```python
from build123d import *

# Parameters (mm, degrees)
SKETCH1_R           = 2.65
SKETCH1_W           = 1
SKETCH1_H           = 8
SKETCH1_W_2         = 14
BOSS_EXTRUDE1_DEPTH = 5
CHAMFER1_SIZE       = 3
BOSS_EXTRUDE2_DEPTH = 4
SKETCH3_R           = 5
CUT_EXTRUDE1_DEPTH  = 11.5


with BuildPart() as part:
    # Sketch1 → Boss-Extrude1 (new body)
    with BuildSketch(Plane.XY):
        Polygon((-14, -2.5), (-14, 0), (-15, 0), (-15, 8), (-14, 8), (-14, 10.5), (-27.5, 10.5), (-27.5, -2.5), align=None)
        with Locations((-21, 4)):
            Circle(SKETCH1_R, mode=Mode.SUBTRACT)
        with Locations((-14.5, 4)):
            Rectangle(SKETCH1_W, SKETCH1_H)
        with Locations((-7, 4)):
            Rectangle(SKETCH1_W_2, SKETCH1_H)
        with Locations((7, 4)):
            Rectangle(SKETCH1_W_2, SKETCH1_H)
        with Locations((14.5, 4)):
            Rectangle(SKETCH1_W, SKETCH1_H)
        Polygon((15, 8), (15, 0), (14, 0), (14, -2.5), (27.5, -2.5), (27.5, 10.5), (14, 10.5), (14, 8), align=None)
        with Locations((21, 4)):
            Circle(SKETCH1_R, mode=Mode.SUBTRACT)
    extrude(amount=BOSS_EXTRUDE1_DEPTH)

    # Chamfer1
    chamfer1_edges = [part.edges().sort_by_distance(p)[0] for p in [
        (27.5, 10.5, 2.5),
        (27.5, -2.5, 2.5),
        (-27.5, -2.5, 2.5),
        (-27.5, 10.5, 2.5),
    ]]
    chamfer(chamfer1_edges, length=CHAMFER1_SIZE)

    # Sketch2 → Boss-Extrude2 (add, symmetric)
    with BuildSketch(Plane(origin=(0, 4, 0), x_dir=(1, 0, 0), z_dir=(0, 1, 0))):
        with BuildLine():
            Line((-14, -5), (-14, 10))
            ThreePointArc((-14, 10), (0, 24), (14, 10))
            Line((14, 10), (14, -5))
            Line((14, -5), (-14, -5))
        make_face()
    extrude(amount=BOSS_EXTRUDE2_DEPTH, both=True)

    # Sketch3 → Cut-Extrude1 (cut, through all)
    with BuildSketch(Plane(origin=(0, 8, 0), x_dir=(1, 0, 0), z_dir=(0, 1, 0))):
        with Locations((0, 10)):
            Circle(SKETCH3_R)
    extrude(amount=-CUT_EXTRUDE1_DEPTH, mode=Mode.SUBTRACT)


solid = part.part
```
For this review, take the finished solid that the model builds, in its own axes (mm). A direction names the side the tool comes from. Give positions to 0.01 mm unless a question says otherwise; leave off trailing zeros. Write each loop counter-clockwise with the first axis right and the second up, starting at its lowest first coordinate (ties: lowest second). Pieces come first, ordered by that corner, then holes. Notation, with made-up numbers: M 52,-5.75 L 101,-5.75 A30 ccw 101,32.25 Z; hole C 49,35.5 d11. An arc over 180 degrees is marked long. One line per item, written item: value.
1) For P1, Ø6.5, axis at y = 3, z = -5.5, coming from the -X side; P2, Ø12, axis at x = 8, z = -2.5, coming from the +Y side; P3, Ø1.5, axis at y = -0.5, z = -1, coming from the +X side; P4, Ø1, axis at y = 9, z = -2, coming from the -X side, all flat-tipped, find the tip position at first contact; note any pin that passes through.
Results are:
P1: stops at x = -14
P2: stops at y = 8
P3: stops at x = 14
P4: passes through
2) Take a section at D-D, the plane x = 21. Write out the cut boundary in (y, z).
Results are:
outline: M -2.5,0 L 1.35,0 L 1.35,5 L -2.5,5 Z; M 6.65,0 L 10.5,0 L 10.5,5 L 6.65,5 Z
3) Take a section at A-A, the plane x = 0. Write out the cut boundary in (y, z).
Results are:
outline: M 0,-24 L 8,-24 L 8,-15 L 0,-15 Z; M 0,-5 L 8,-5 L 8,5 L 0,5 Z
4) Take a section at C-C, the plane z = 1. Write out the cut boundary in (x, y), then the cut area to 3 significant figures.
Results are:
outline: M -27.5,0.5 L -24.5,-2.5 L -14,-2.5 L -14,0 L 14,0 L 14,-2.5 L 24.5,-2.5 L 27.5,0.5 L 27.5,7.5 L 24.5,10.5 L 14,10.5 L 14,8 L -14,8 L -14,10.5 L -24.5,10.5 L -27.5,7.5 Z; hole C -21,4 d5.3; hole C 21,4 d5.3
area: 513 mm²
5) Take a section at B-B, the plane y = 2.5. Write out the cut boundary in (x, z), then the cut area to 3 significant figures.
Results are:
outline: M -27.5,0 L -23.18,0 L -23.18,5 L -27.5,5 Z; M -18.82,0 L -14,0 L -14,-10 A14 ccw 14,-10 L 14,0 L 18.82,0 L 18.82,5 L -18.82,5 Z; M 23.18,0 L 27.5,0 L 27.5,5 L 23.18,5 Z; hole C 0,-10 d10
area: 741 mm²
6) For faces 1 (the flat face through (0, 0, -3)), 2 (the flat face through (18, 4, 0)), 3 (the flat face through (0, 8, -3)), list the 3-axis set-ups (+Z, -Z, +X, -X, +Y, -Y) from which the entire face can be reached by the end or side of a thin tool; tool diameter is ignored.
Results are:
face 1: +Z, -Z, -Y
face 2: -Z, +X, +Y, -Y
face 3: +Z, -Z, +Y
7) The part is to be moulded in two halves that separate along Y. For faces 4 (the flat face through (-26, -1, 2)), 5 (the flat face through (-14, -1, 2)), 6 (the cylindrical face through (23.45, 2.99, 2.46)), 7 (the cylindrical face through (-18.55, 2.99, 2.46)), say which applies: +Y half, -Y half, draft (parallel to the pull), parting line (faces both ways), or undercut.
Results are:
face 4: -Y half
face 5: draft
face 6: undercut
face 7: undercut
8) For line 1 (Z direction, x = 0, y = 5); line 2 (Y direction, x = 21, z = 1.75); line 3 (X direction, y = 6, z = -10), list the stretches that pass through material, from the lowest coordinate up. Write a range as from..to.
Results are:
line 1: z = -24..-15, -5..5
line 2: y = -2.5..1.35, 6.65..10.5
line 3: x = -14..-5, 5..14
